Job drawing, mm, ordinate dimensions from the low corner. One solid piece. A direction names the side the tool comes from. Give positions to 0.01 mm unless a question says otherwise; leave off trailing zeros. Order: outer loops, then holes, each group sorted by start corner. A loop starts at its lowest first (then second) coordinate and runs counter-clockwise, first axis right, second up.
1. Slice it at C-C on x = 6. List the corners of the cut face in (y, z), and give its area (3 significant figures).
2. Which spindle directions (+Z, -Z, +X, -X, +Y, -Y) get a long thin tool onto all of the face, cutting with end or side? Do the marked faces 5 and 6. Say none if no direction does.
3. Probe line 1 (Y direction, x = 55.75, z = 11.05); line 2 (X direction, y = 12, z = 12.25); line 3 (Y direction, x = 23, z = 10.25). List the from-to ranges inside material, lowest first.
4. Slice it at A-A on z = 10.75. Give the number of separate pieces and of enclosed holes in the cut face, and give its area (3 significant figures).
5. Slice it at D-D on x = 32. List the corners of the cut face in (y, z), and give its area (3 significant figures).
6. Slice it at B-B on x = 23.95. List the corners of the cut face in (y, z), and give its area (3 significant figures).
7. Mould opens along X. For the marked faces 1, 2, 3 and 4 say: +X half, -X half, draft (parallel to the pull), parting line (faces both ways), or undercut.
8. Drop flat-ended pins along their axis: pin 1 Ø2 at (x, y) = (39.5, 8) entering from +Z; pin 2 Ø1.5 at (x, z) = (15.5, 7.5) entering from -Y. Give the stop position or say it passes through.
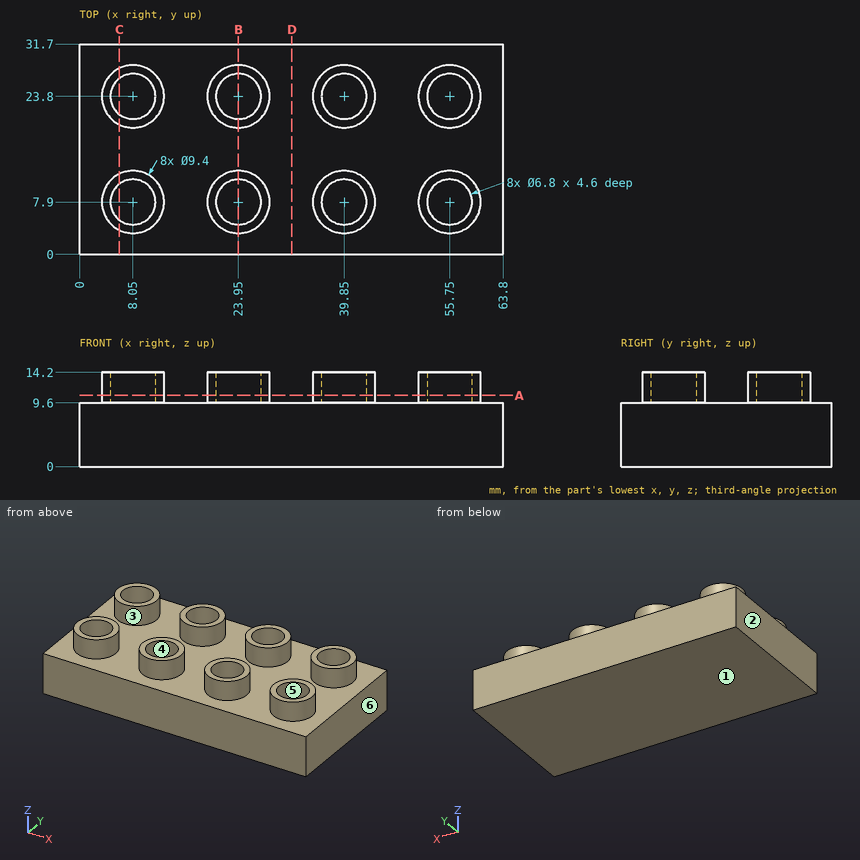
Data:
1. outline: (0, 0) - (31.7, 0) - (31.7, 9.6) - (28.03, 9.6) - (28.03, 14.2) - (26.51, 14.2) - (26.51, 9.6) - (21.09, 9.6) - (21.09, 14.2) - (19.57, 14.2) - (19.57, 9.6) - (12.13, 9.6) - (12.13, 14.2) - (10.61, 14.2) - (10.61, 9.6) - (5.19, 9.6) - (5.19, 14.2) - (3.67, 14.2) - (3.67, 9.6) - (0, 9.6) - close
1. area: 332 mm2
2. face 5: +Z
2. face 6: +Z, -Z, +X, +Y, -Y
3. line 1: y = 3.2 to 4.5, 11.3 to 12.6, 19.1 to 20.4, 27.2 to 28.5
3. line 2: x = 5.75 to 10.35, 21.65 to 26.25, 37.55 to 42.15, 53.45 to 58.05
3. line 3: y = 3.3 to 4.64, 11.16 to 12.5, 19.2 to 20.54, 27.06 to 28.4
4. separate pieces: 8
4. enclosed holes: 8
4. area: 265 mm2
5. outline: (0, 0) - (31.7, 0) - (31.7, 9.6) - (0, 9.6) - close
5. area: 304 mm2
6. outline: (0, 0) - (31.7, 0) - (31.7, 9.6) - (28.5, 9.6) - (28.5, 14.2) - (27.2, 14.2) - (27.2, 9.6) - (20.4, 9.6) - (20.4, 14.2) - (19.1, 14.2) - (19.1, 9.6) - (12.6, 9.6) - (12.6, 14.2) - (11.3, 14.2) - (11.3, 9.6) - (4.5, 9.6) - (4.5, 14.2) - (3.2, 14.2) - (3.2, 9.6) - (0, 9.6) - close
6. area: 328 mm2
7. face 1: draft
7. face 2: -X half
7. face 3: undercut
7. face 4: undercut
8. pin 1: stops at z = 9.6
8. pin 2: stops at y = 0
